```python
from build123d import *

# Parameters (mm, degrees)
SKETCH9_R           = 13.081
BOSS_EXTRUDE2_DEPTH = 177.8
SKETCH3_R           = 9.906
CUT_EXTRUDE1_DEPTH  = 171.45
CUT_EXTRUDE2_DEPTH  = 206.013596075


with BuildPart() as part:
    # Sketch9 → Boss-Extrude2 (new body)
    with BuildSketch(Plane(origin=(0, 0, 0), x_dir=(1, 0, 0), z_dir=(0, 0.7071067811865464, 0.7071067811865487))):
        with Locations(Location((0, 0, 0), (0, 0, 90))):
            Circle(SKETCH9_R)
    extrude(amount=BOSS_EXTRUDE2_DEPTH)

    # Sketch3 → Cut-Extrude1 (cut)
    with BuildSketch(Plane(origin=(0, 429.24717139, -177.8), x_dir=(1, 0, 0), z_dir=(0, -0.7071067811865464, -0.7071067811865487))):
        with Locations(Location((0, 429.24717139, 0), (0, 0, 270))):
            Circle(SKETCH3_R)
    extrude(amount=CUT_EXTRUDE1_DEPTH, mode=Mode.SUBTRACT)

    # Sketch5 → Cut-Extrude2 (cut, through all)
    with BuildSketch(Plane(origin=(0, 52.076414305, -52.076414305), x_dir=(-1, 0, 0), z_dir=(0, -0.7071067811865464, -0.7071067811865487))):
        with BuildLine():
            Line((-1.524, -64.94767139), (1.524, -64.94767139))
            Line((1.524, -64.94767139), (1.524, -68.867768054))
            ThreePointArc((1.524, -68.867768054), (5.0165, -73.64717139), (1.524, -78.426574726))
            Line((1.524, -78.426574726), (1.524, -82.34667139))
            Line((1.524, -82.34667139), (-1.524, -82.34667139))
            Line((-1.524, -82.34667139), (-1.524, -78.426574726))
            ThreePointArc((-1.524, -78.426574726), (-5.0165, -73.64717139), (-1.524, -68.867768054))
            Line((-1.524, -68.867768054), (-1.524, -64.94767139))
        make_face()
    extrude(amount=-CUT_EXTRUDE2_DEPTH, mode=Mode.SUBTRACT)


solid = part.part
```
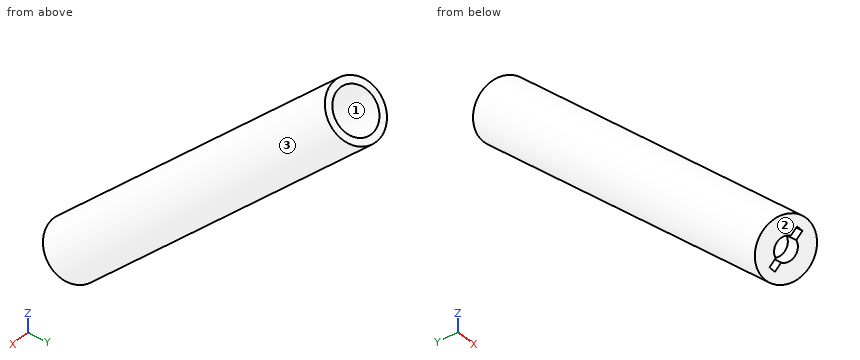
Can you work these out from the model? Positions are in its coordinate system, mm. Face numbers are marked on the shaded views. Coordinates: 2 decimals unless noted, no trailing zeros. Loops run counter-clockwise (first coordinate to the right, second up) from the corner with the lowest first, then second, coordinate; pieces in that order, holes last. Notation, with made-up numbers: (4.5, 75.5) -> (44.5, 75.5) arc R19 cw to (44.5, 108.5) -> close; hole circle Ø2 at (-2.5, 20.25). An arc over 180 degrees is marked (long way). Put each result on its own line as item: value. Start each with the question number.
Q1. If I drill on line 1 (X direction, y = 59.5, z = 59); line 2 (Y direction, x = -2, z = 105); line 3 (Z direction, x = -0.25, y = 106.5), over which ranges is the centre line in solid material (lowest first)? Write a range as [from, to].
Q2. I want a section at A-A (x = -6.75). Write out the boundary of the cut face in (y, z), plus the area to 3 significant figures.
Q3. Thinking about a two-plate mould opening in Y: for the marked faces 1, 2 and 3, which applies, pulls with the +Y half, pulls with the -Y half, needs draft (parallel to the pull), parting line crosses it, or undercut?
Q4. I'm going to push flat-ended pins straight in: P1, Ø6, axis at x = 5.5, z = 81.5, coming from the -Y side; P2, Ø8, axis at y = 6, z = -1, coming from the -X side; P3, Ø6, axis at y = -3, z = 8, coming from the +X side; P4, Ø12, axis at y = 115.5, z = 118.5, coming from the +X side. Where does each tip first touch, or does it pass through?
Taken from the geometry:
1. line 1: x = [-13.08, -9.9], [9.9, 13.08]
1. line 2: y = [86.72, 91.28], [118.72, 123.28]
1. line 3: z = [88, 92.5], [120.5, 125]
2. outline: (-7.92, 7.92) -> (7.92, -7.92) -> (133.65, 117.8) -> (130.85, 120.6) -> (9.62, -0.64) -> (-0.64, 9.62) -> (120.6, 130.85) -> (117.8, 133.65) -> close
2. area: 1,500 mm2
3. face 1: undercut
3. face 2: pulls with the -Y half
3. face 3: parting line crosses it
4. P1: stops at y = 61.28
4. P2: stops at x = -13.05
4. P3: stops at x = 12.18
4. P4: stops at x = 13.08
